Could you check a few things on this model? Use its own coordinates, in mm. Round coordinates to 2 decimals unless told otherwise and drop trailing zeros. Loops run counter-clockwise (first coordinate to the right, second up) from the corner with the lowest first, then second, coordinate; pieces in that order, holes last. Notation, with made-up numbers: (-14, -2.75) -> (4, -2.75) arc R23 ccw to (4, 31.25) -> close; hole circle Ø11 at (89.25, -38). An arc over 180 degrees is marked (long way). Write each question's results on one line, items separated by ' | '.
from build123d import *

# Parameters (mm, degrees)
F1_DEPTH = 70
F4_DEPTH = 20
F6_DEPTH = 15
F7_W     = 6
F7_H     = 2
F8_DEPTH = 5


with BuildPart() as f1:
    # F0 (on Front) → F1 (new body)
    with BuildSketch(Plane.XZ):
        with BuildLine():
            Line((-0.5, 2.5), (-0.5, 1.9364916731))
            ThreePointArc((-0.5, 1.9364916731), (0, -2), (0.5, 1.9364916731))
            Line((0.5, 1.9364916731), (0.5, 2.5))
            Line((0.5, 2.5), (-0.5, 2.5))
        make_face()
    extrude(amount=F1_DEPTH)

    # F3 (on offset) → F4 (cut)
    with BuildSketch(Plane.XZ.offset(60)):
        with BuildLine():
            ThreePointArc((-0.5, 1.9364916731), (0.0006379585, 1.9999998983), (0.5012352994, 1.9361722998))
            Line((0.5012352994, 1.9361722998), (0.5, 2.5))
            Line((0.5, 2.5), (-0.5, 2.5))
            Line((-0.5, 2.5), (-0.5, 1.9364916731))
        make_face()
    extrude(amount=-F4_DEPTH, mode=Mode.SUBTRACT)

    # F5 (on face) → F6 (cut)
    with BuildSketch(Plane(origin=(0, 0, 0), x_dir=(-1, 0, 0), z_dir=(0, 1, 0))):
        with BuildLine():
            Line((-0.5, 2.5), (-0.5, 1.9364916731))
            ThreePointArc((-0.5, 1.9364916731), (0, 2), (0.5, 1.9364916731))
            Line((0.5, 1.9364916731), (0.5, 2.5))
            Line((0.5, 2.5), (-0.5, 2.5))
        make_face()
    extrude(amount=-F6_DEPTH, mode=Mode.SUBTRACT)

    # F7 (on face) → F8 (cut)
    with BuildSketch(Plane(origin=(0, 0, 0), x_dir=(-1, 0, 0), z_dir=(0, 1, 0))):
        Rectangle(F7_W, F7_H)
    extrude(amount=-F8_DEPTH, mode=Mode.SUBTRACT)


solid = f1.part
1) I want a section at C-C, the plane y = -57. Write out the boundary of the cut face in (x, z).
Model answer:
outline: circle Ø4 at (0, 0)
2) I want a section at B-B, the plane z = 0. Write out the boundary of the cut face in (x, y).
Model answer:
outline: (-2, -70) -> (2, -70) -> (2, -5) -> (-2, -5) -> close
3) I want a section at A-A, the plane y = -38.5. Write out the boundary of the cut face in (x, z).
Model answer:
outline: (-0.5, 1.94) arc R2 ccw (long way) to (0.5, 1.94) -> (0.5, 2.5) -> (-0.5, 2.5) -> close
4) If we mould it in two halves opening along Z, with no side actions, what happens to faces 1 (the flat face through (0, -70, 0)), 2 (the flat face through (0, -5, 0))? For each: released by +Z, released by -Z, zero draft, split by the parting line, or undercut.
Model answer:
face 1: zero draft | face 2: undercut
5) I'm going to push flat-ended pins straight in: pin 1 (1 mm diameter, centred on x = 1.5, y = -53.5, fed in from +Z); pin 2 (1.7 mm diameter, centred on x = -0.5, y = -3.5, fed in from -Z); pin 3 (0.6 mm diameter, centred on y = -65, z = 2, fed in from -X); pin 4 (0.6 mm diameter, centred on x = 0.5, z = 0, fed in from +Y). Where does each tip first touch, or does it pass through?
Model answer:
pin 1: stops at z = 1.73 | pin 2: stops at z = -2 | pin 3: stops at x = -1.05 | pin 4: stops at y = -5
6) I need wall thicknesses on line 1 (Z direction, x = -0.1, y = -44); line 2 (Z direction, x = 1, y = -57.5); line 3 (Y direction, x = 0.05, z = -0.3). Which ranges of each line are inside material? Lowest first, please.
Model answer:
line 1: z = -2 to 2 | line 2: z = -1.73 to 1.73 | line 3: y = -70 to -5
